```python
from build123d import *

# Parameters (mm, degrees)
CYLINDER015_R     = 1
CYLINDER015_DEPTH = 3
CYLINDER014_R     = 1
CYLINDER014_DEPTH = 3
CYLINDER013_R     = 1
CYLINDER013_DEPTH = 3
CYLINDER016_R     = 1
CYLINDER016_DEPTH = 3
BOX004_W          = 26
BOX004_H          = 17.1
BOX004_DEPTH      = 2
BOX005_W          = 32
BOX005_H          = 8
BOX005_DEPTH      = 2
FILLET003_R       = 1


with BuildPart() as cilindro015:
    # Cylinder015 → Cylinder015 (new body)
    with BuildSketch(Plane(origin=(89.75, 253.65, 4), x_dir=(1, 0, 0), z_dir=(0, 0, 1))):
        Circle(CYLINDER015_R)
    extrude(amount=CYLINDER015_DEPTH)


with BuildPart() as cilindro014:
    # Cylinder014 → Cylinder014 (new body)
    with BuildSketch(Plane(origin=(89.75, 240.65, 4), x_dir=(1, 0, 0), z_dir=(0, 0, 1))):
        Circle(CYLINDER014_R)
    extrude(amount=CYLINDER014_DEPTH)


with BuildPart() as cilindro013:
    # Cylinder013 → Cylinder013 (new body)
    with BuildSketch(Plane(origin=(110.85, 240.65, 4), x_dir=(1, 0, 0), z_dir=(0, 0, 1))):
        Circle(CYLINDER013_R)
    extrude(amount=CYLINDER013_DEPTH)


with BuildPart() as fusion011:
    # Cylinder016 → Cylinder016 (new body)
    with BuildSketch(Plane(origin=(110.85, 253.65, 4), x_dir=(1, 0, 0), z_dir=(0, 0, 1))):
        Circle(CYLINDER016_R)
    extrude(amount=CYLINDER016_DEPTH)

    # Fusion011: union Cilindro015, Cilindro014, Cilindro013
    add(cilindro015.part)
    add(cilindro014.part)
    add(cilindro013.part)


with BuildPart() as fusion011_1:
    # Fusion011 placement: moved
    add(fusion011.part.moved(Location((0, 0, -4))))


with BuildPart() as cubo004:
    # Box004 → Box004 (new body)
    with BuildSketch(Plane(origin=(87.15, 238.8, -2), x_dir=(1, 0, 0), z_dir=(0, 0, 1))):
        with Locations((13, 8.55)):
            Rectangle(BOX004_W, BOX004_H)
    extrude(amount=BOX004_DEPTH)


with BuildPart() as tapa:
    # Box005 → Box005 (new body)
    with BuildSketch(Plane(origin=(84, 247.5, -2), x_dir=(1, 0, 0), z_dir=(0, 0, 1))):
        with Locations((16, 4)):
            Rectangle(BOX005_W, BOX005_H)
    extrude(amount=BOX005_DEPTH)

    # Fusion016: union Cubo004
    add(cubo004.part)

    # Fusion017: union Fusion011
    add(fusion011_1.part)


with BuildPart() as tapa_1:
    # Fusion017 placement: moved
    add(tapa.part.moved(Location((0, 0, -26))))

    # Fillet003
    fillet003_edges = [tapa_1.edges().sort_by_distance(p)[0] for p in [
        (109.85, 253.65, -26),
        (109.85, 240.65, -26),
        (88.75, 240.65, -26),
        (88.75, 253.65, -26),
    ]]
    fillet(fillet003_edges, radius=FILLET003_R)


solid = tapa_1.part
```
Read the model definition and answer for the solid it produces. Units are mm, in the model's axes. A direction names the side the tool comes from. Coordinates: 2 decimals unless noted, no trailing zeros. Write each loop counter-clockwise with the first axis right and the second up, starting at its lowest first coordinate (ties: lowest second). Pieces come first, ordered by that corner, then holes. Notation, with made-up numbers: (-2.75, 3) - (18.25, 3) arc R18 ccw to (18.25, 34) - close; hole circle Ø2 at (20, -14). An arc over 180 degrees is marked (long way). Answer as a JSON object with one key per item and string values. Group by question number.
1. A cutting plane is placed at A-A (y = 240.65). Determine the outline of the cut face in (x, z).
2. The mould has two halves that part along X. Classify faces 1 (the flat face through (87.15, 243, -27)), 2 (the flat face through (86, 255.5, -27)), 3 (the cylindrical face through (110.633, 239.674, -24.022)): +X half, -X half, draft (parallel to the pull), parting line (faces both ways), or undercut.
3. Consider L1, parallel to X at y = 240, z = -24.4; L2, parallel to Z at x = 114, y = 250.25; L3, parallel to X at y = 247.25, z = -27. Determine where each line is inside the solid, lowest interval first. Write a range as [from, to].
4. Which of the six approach directions +Z, -Z, +X, -X, +Y, -Y give full straight-line access (tool end or side, diameter ignored) to faces 4 (the flat face through (86, 247.5, -27)), 5 (the flat face through (115, 247.5, -27)), 6 (the cylindrical face through (89.533, 239.674, -24.022))?
5. Each of these flat-tipped pins is pushed along its axis until it touches: P1, Ø1.6, axis at x = 114, z = -27, coming from the +Y side; P2, Ø5, axis at x = 100.5, y = 244.5, coming from the +Z side; P3, Ø3, axis at y = 244, z = -25.5, coming from the +X side; P4, Ø1.5, axis at x = 98.5, z = -24, coming from the +Y side. Where does it stop, or does it pass through?
6. A cutting plane is placed at B-B (y = 253.65). Determine the outline of the cut face in (x, z), plus the area to 3 significant figures.
7. A cutting plane is placed at C-C (x = 102.5). Determine the outline of the cut face in (y, z), plus the area to 3 significant figures.
8. A cutting plane is placed at D-D (y = 248). Determine the outline of the cut face in (x, z), plus the area to 3 significant figures.
Worked out:
{
 "1": {"outline": "(87.15, -28) - (113.15, -28) - (113.15, -26) - (112.85, -26) arc R1 cw to (111.85, -25) - (111.85, -23) - (109.85, -23) - (109.85, -25) arc R1 cw to (108.85, -26) - (91.75, -26) arc R1 cw to (90.75, -25) - (90.75, -23) - (88.75, -23) - (88.75, -25) arc R1 cw to (87.75, -26) - (87.15, -26) - close"},
 "2": {"face 1": "-X half", "face 2": "draft", "face 3": "undercut"},
 "3": {"L1": "x = [88.99, 90.51], [110.09, 111.61]", "L2": "z = [-28, -26]", "L3": "x = [87.15, 113.15]"},
 "4": {"face 4": "+Z, -Z, -X, -Y", "face 5": "+Z, -Z, +X, -Y", "face 6": "+Z"},
 "5": {"P1": "stops at y = 255.5", "P2": "stops at z = -26", "P3": "stops at x = 113.15", "P4": "passes through"},
 "6": {"outline": "(84, -28) - (116, -28) - (116, -26) - (112.85, -26) arc R1 cw to (111.85, -25) - (111.85, -23) - (109.85, -23) - (109.85, -25) arc R1 cw to (108.85, -26) - (91.75, -26) arc R1 cw to (90.75, -25) - (90.75, -23) - (88.75, -23) - (88.75, -25) arc R1 cw to (87.75, -26) - (84, -26) - close", "area": "76.9 mm²"},
 "7": {"outline": "(238.8, -28) - (255.9, -28) - (255.9, -26) - (238.8, -26) - close", "area": "34.2 mm²"},
 "8": {"outline": "(84, -28) - (116, -28) - (116, -26) - (84, -26) - close", "area": "64.0 mm²"}
}
